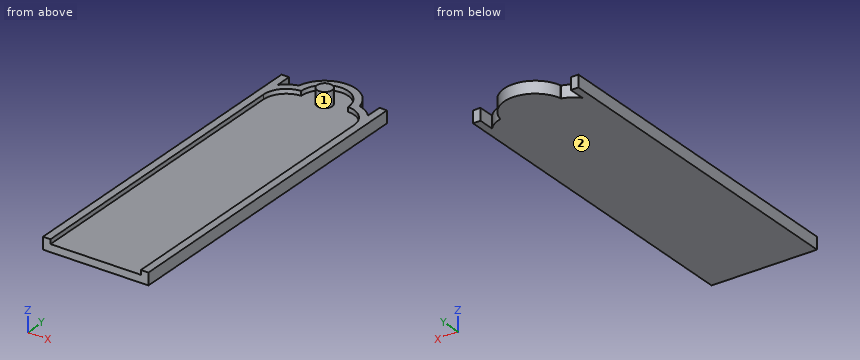
from build123d import *

# Parameters (mm, degrees)
SKETCH2_R           = 50
BOSS_EXTRUDE3_DEPTH = 50
BOSS_EXTRUDE4_DEPTH = 80
SKETCH2_9_R         = 50
SKETCH2_9_R_2       = 20
BOSS_EXTRUDE5_DEPTH = 150


with BuildPart() as part:
    # Sketch2 → Boss-Extrude3 (new body)
    with BuildSketch(Plane.XY):
        with BuildLine():
            Line((-283.78190134, 487.937190165), (-283.78190134, -1512.062809835))
            Line((-283.78190134, -1512.062809835), (316.21809866, -1512.062809835))
            Line((316.21809866, -1512.062809835), (316.21809866, 487.937190165))
            ThreePointArc((316.21809866, 487.937190165), (274.438439922, 591.804209653), (172.37332883, 637.810847428))
            ThreePointArc((172.37332883, 637.810847428), (169.296362007, 637.905601155), (166.21809866, 637.937190165))
            Line((166.21809866, 637.937190165), (172.373379941, 637.937190165))
            ThreePointArc((172.373379941, 637.937190165), (16.21809866, 794.092471446), (-139.937182621, 637.937190165))
            Line((-139.937182621, 637.937190165), (-139.660119377, 637.937190165))
            Line((-139.660119377, 637.937190165), (-133.78190134, 637.937190165))
            ThreePointArc((-133.78190134, 637.937190165), (-136.860164687, 637.905601155), (-139.93713151, 637.810847428))
            ThreePointArc((-139.93713151, 637.810847428), (-242.002242601, 591.804209653), (-283.78190134, 487.937190165))
        make_face()
        with Locations((16.21809866, 637.937190165)):
            Circle(SKETCH2_R, mode=Mode.SUBTRACT)
    extrude(amount=BOSS_EXTRUDE3_DEPTH)

    # Sketch2_8 → Boss-Extrude4 (add)
    with BuildSketch(Plane.XY):
        with BuildLine():
            Line((-333.78190134, 487.937190165), (-333.78190134, -1512.062809835))
            Line((-333.78190134, -1512.062809835), (-283.78190134, -1512.062809835))
            Line((-283.78190134, -1512.062809835), (-283.78190134, 487.937190165))
            ThreePointArc((-283.78190134, 487.937190165), (-242.002242601, 591.804209653), (-139.93713151, 637.810847428))
            ThreePointArc((-139.93713151, 637.810847428), (-139.937169843, 637.874018792), (-139.937182621, 637.937190165))
            ThreePointArc((-139.937182621, 637.937190165), (16.21809866, 794.092471446), (172.373379941, 637.937190165))
            ThreePointArc((172.373379941, 637.937190165), (172.373367163, 637.874018792), (172.37332883, 637.810847428))
            ThreePointArc((172.37332883, 637.810847428), (274.438439922, 591.804209653), (316.21809866, 487.937190165))
            Line((316.21809866, 487.937190165), (316.21809866, -1512.062809835))
            Line((316.21809866, -1512.062809835), (366.21809866, -1512.062809835))
            Line((366.21809866, -1512.062809835), (366.21809866, 487.937190165))
            Line((366.21809866, 487.937190165), (366.21809866, 727.937190165))
            Line((366.21809866, 727.937190165), (316.21809866, 727.937190165))
            Line((316.21809866, 727.937190165), (316.21809866, 620.224755718))
            ThreePointArc((316.21809866, 620.224755718), (271.509827539, 657.977337865), (217.788355507, 681.174113678))
            ThreePointArc((217.788355507, 681.174113678), (19.689586458, 844.063240853), (-183.78190134, 687.937190165))
            Line((-183.78190134, 687.937190165), (-183.78190134, 681.586357475))
            ThreePointArc((-183.78190134, 681.586357475), (-184.567448055, 681.381828873), (-185.352158186, 681.174113678))
            ThreePointArc((-185.352158186, 681.174113678), (-239.073630218, 657.977337865), (-283.78190134, 620.224755718))
            Line((-283.78190134, 620.224755718), (-283.78190134, 727.937190165))
            Line((-283.78190134, 727.937190165), (-333.78190134, 727.937190165))
            Line((-333.78190134, 727.937190165), (-333.78190134, 487.937190165))
        make_face()
    extrude(amount=BOSS_EXTRUDE4_DEPTH)

    # Sketch2_9 → Boss-Extrude5 (add)
    with BuildSketch(Plane.XY):
        with Locations((16.21809866, 637.937190165)):
            Circle(SKETCH2_9_R)
        with Locations((16.21809866, 637.937190165)):
            Circle(SKETCH2_9_R_2, mode=Mode.SUBTRACT)
        with Locations((16.21809866, 637.937190165)):
            Circle(SKETCH2_9_R_2)
    extrude(amount=BOSS_EXTRUDE5_DEPTH)


solid = part.part
Check sheet for the modelled part. Datum: model origin and axes. Units: mm. Face numbers are marked on the shaded views. Round coordinates to 2 decimals unless told otherwise and drop trailing zeros. Order: outer loops, then holes, each group sorted by start corner. A loop starts at its lowest first (then second) coordinate and runs counter-clockwise, first axis right, second up.
(1) Cross-section at D-D, the plane z = 114. Enter the section's corners in (x, y).
(2) Cross-section at C-C, the plane x = -214.5. Enter the section's corners in (y, z).
(3) Go/stop test with flat-tipped pins: P1, Ø8, axis at x = 95, z = 68, coming from the +Y side; P2, Ø2, axis at x = -100, y = -1106.5, coming from the +Z side. Record where each tip stops, or that it passes through.
(4) Cross-section at B-B, the plane y = -277.5. Enter the section's corners in (x, z).
(5) Scan lines: probe 1 along X at (y, z) = (-954, 58); probe 2 along Z at (x, y) = (294, -351.5); probe 3 along Y at (x, z) = (22, 31). Record each from-to range of solid material in increasing order.
(6) Draft check along Y on the marked faces 1 and 2. Enter one of: pulls with the +Y half, pulls with the -Y half, needs draft (parallel to the pull), parting line crosses it, or undercut.
Check sheet entries:
1. outline: circle Ø100 at (16.22, 637.94)
2. outline: (-1512.06, 0) - (670.93, 0) - (670.93, 80) - (614.37, 80) - (614.37, 50) - (-1512.06, 50) - close
3. P1: stops at y = 830.05
3. P2: stops at z = 50
4. outline: (-333.78, 0) - (366.22, 0) - (366.22, 80) - (316.22, 80) - (316.22, 50) - (-283.78, 50) - (-283.78, 80) - (-333.78, 80) - close
5. probe 1: x = -333.78 to -283.78, 316.22 to 366.22
5. probe 2: z = 0 to 50
5. probe 3: y = -1512.06 to 844.01
6. face 1: undercut
6. face 2: needs draft
